The drawing under review shows one solid part. Ordinate dimensions are in mm from its lowest x, y, z. Coordinates: 2 decimals unless noted, no trailing zeros. Write each loop counter-clockwise with the first axis right and the second up, starting at its lowest first coordinate (ties: lowest second). Pieces come first, ordered by that corner, then holes. Notation, with made-up numbers: (35, 19) -> (53, 19) arc R6 ccw to (53, 29) -> close; hole circle Ø7 at (4, 54.5). An arc over 180 degrees is marked (long way). One line per item, written item: value. Start each with the question number.
1) Add section A-A (y = 107.5). State the section outline as (x, z) points.
2) Mouldability with a two-part tool opening along X and no side actions: class the marked faces 1 and 2 as released by +X, released by -X, zero draft, split by the parting line, or undercut.
3) Add section B-B (x = 25). State the section outline as (y, z) points, and give its area (3 significant figures).
4) For probe 1 along X at (y, z) = (107.5, 1.5); probe 2 along Y at (x, z) = (25.5, 6.25); probe 3 along Y at (x, z) = (23.5, 2.5), list the stretches that pass through material, from the lowest coordinate up. Write a range as from..to.
5) For pin 1 Ø21 at (x, y) = (25, 107.5) entering from -Z, flat-tipped, find the tip position at first contact; note if it passes through.
6) Add section C-C (z = 1.25). State the section outline as (x, y) points, and give its area (3 significant figures).
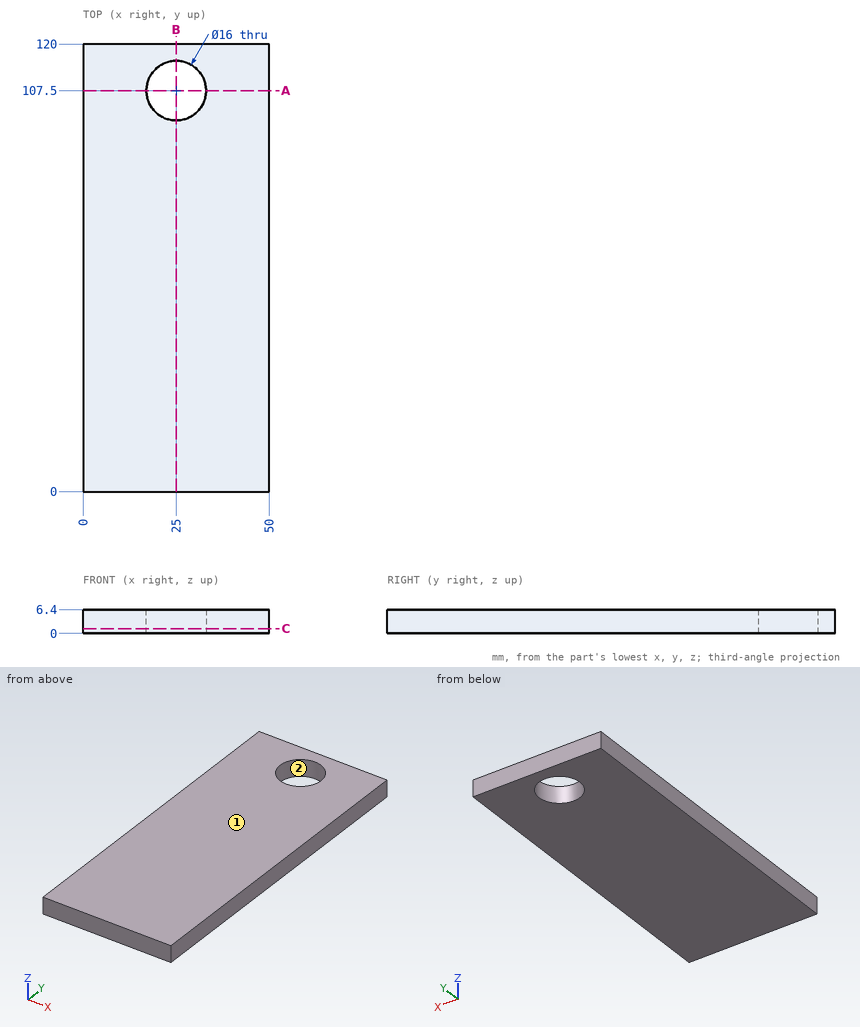
Numbers:
1. outline: (0, 0) -> (17, 0) -> (17, 6.4) -> (0, 6.4) -> close; (33, 0) -> (50, 0) -> (50, 6.4) -> (33, 6.4) -> close
2. face 1: zero draft
2. face 2: undercut
3. outline: (0, 0) -> (99.5, 0) -> (99.5, 6.4) -> (0, 6.4) -> close; (115.5, 0) -> (120, 0) -> (120, 6.4) -> (115.5, 6.4) -> close
3. area: 666 mm²
4. probe 1: 0..17, 33..50
4. probe 2: 0..99.52, 115.48..120
4. probe 3: 0..99.64, 115.36..120
5. pin 1: z = 0
6. outline: (0, 0) -> (50, 0) -> (50, 120) -> (0, 120) -> close; hole circle Ø16 at (25, 107.5)
6. area: 5,800 mm²
